The listing builds one solid part. Answer for the finished solid, in the listing's coordinates (mm). Give positions to 0.01 mm unless a question says otherwise; leave off trailing zeros. Loops run counter-clockwise (first coordinate to the right, second up) from the corner with the lowest first, then second, coordinate; pieces in that order, holes last. Notation, with made-up numbers: (51, 25.5) - (78, 25.5) arc R27 cw to (78, 43.5) - close; hole circle Ø1 at (66, 22.25). An arc over 180 degrees is marked (long way). Answer in a Markdown table with one row per item. Add a question column.
```python
from build123d import *

# Parameters (mm, degrees)
SKETCH1_W           = 456
SKETCH1_H           = 626
BASE_FLANGE1_DEPTH  = 1
SKETCH6_W           = 130
SKETCH6_H           = 60
BOSS_EXTRUDE1_DEPTH = 10
SKETCH7_W           = 128
SKETCH7_H           = 58
CUT_EXTRUDE2_DEPTH  = 1
SHELL2_START        = -186
SHELL2_OUTLINE_W    = 58
SHELL2_OUTLINE_H    = 8
SHELL2_DEPTH        = 128
FILLET1_R           = 5


# Read off the part's stored shape, not the designer's step: Shell2
# Sheet-metal steps are written as plain solids
with BuildPart() as part:
    # Sketch1 → Base-Flange1 (new body)
    with BuildSketch(Plane.XY):
        Rectangle(SKETCH1_W, SKETCH1_H)
    extrude(amount=-BASE_FLANGE1_DEPTH)

    # Sketch6 → Boss-Extrude1 (add)
    with BuildSketch(Plane.XY):
        with Locations((-122, 254)):
            Rectangle(SKETCH6_W, SKETCH6_H)
    extrude(amount=-BOSS_EXTRUDE1_DEPTH)

    # Sketch7 → Cut-Extrude2 (cut)
    with BuildSketch(Plane.XY):
        with Locations((-122, 254)):
            Rectangle(SKETCH7_W, SKETCH7_H)
    extrude(amount=-CUT_EXTRUDE2_DEPTH, mode=Mode.SUBTRACT)

    # Shell2 outline → Shell2 (cut)
    with BuildSketch(Plane.YZ.offset(SHELL2_START)):
        with Locations((254, -5)):
            Rectangle(SHELL2_OUTLINE_W, SHELL2_OUTLINE_H)
    extrude(amount=SHELL2_DEPTH, mode=Mode.SUBTRACT)

    # Fillet1
    fillet1_edges = [part.edges().sort_by_distance(p)[0] for p in [
        (-57, 284, -5.5),
        (-57, 224, -5.5),
        (-187, 224, -5.5),
        (-187, 284, -5.5),
        (-186, 225, -4.5),
        (-186, 283, -4.5),
        (-58, 283, -4.5),
        (-58, 225, -4.5),
    ]]
    fillet(fillet1_edges, radius=FILLET1_R)


solid = part.part
```
(1) A cutting plane is placed at B-B on x = -156. Determine the outline of the cut face in (y, z).
(2) Find the intervals of material crossed by line 1 along Y through (x, z) = (-111.5, -2.75); line 2 along X through (y, z) = (268, -1.25); line 3 along Z through (x, y) = (193, 231.5), in increasing order. Write a range as [from, to].
(3) The mould has two halves that part along Y. Classify faces 1 (the face through (-123, 254, -9)), 2 (the face through (-3, 4, 0)): pulls with the +Y half, pulls with the -Y half, needs draft (parallel to the pull), parting line crosses it, or undercut.
(4) A cutting plane is placed at A-A on z = -7.5. Determine the outline of the cut face in (x, y), plus the area to 3 significant figures.
(5) A cutting plane is placed at D-D on x = 197.5. Determine the outline of the cut face in (y, z), plus the area to 3 significant figures.
(6) Given pin 1 Ø4.5 at (y, z) = (246, -5) entering from +X; pin 2 Ø4.5 at (y, z) = (253.5, -7) entering from -X; pin 3 Ø4.5 at (x, z) = (-103.5, -4) entering from +Y; pin 4 Ø1 at (x, y) = (69.5, 229.5) entering from +Z, each flat-ended and moving along its own axis, determine where each tip first touches the part or whether it passes through.
(7) A cutting plane is placed at C-C on y = -155.5. Determine the outline of the cut face in (x, z), plus the area to 3 significant figures.
Evaluation:
| question | item | result |
|---|---|---|
| 1 | outline | (-313, -1) - (224, -1) - (224, -10) - (284, -10) - (284, -1) - (313, -1) - (313, 0) - (283, 0) - (283, -9) - (225, -9) - (225, 0) - (-313, 0) - close |
| 2 | line 1 | y = [224, 225], [283, 284] |
| 2 | line 2 | x = [-187, -186], [-58, -57] |
| 2 | line 3 | z = [-1, 0] |
| 3 | face 1 | undercut |
| 3 | face 2 | needs draft |
| 4 | outline | (-187, 229) arc R5 ccw to (-182, 224) - (-62, 224) arc R5 ccw to (-57, 229) - (-57, 279) arc R5 ccw to (-62, 284) - (-182, 284) arc R5 ccw to (-187, 279) - close; hole (-186, 230) arc R5 ccw to (-181, 225) - (-63, 225) arc R5 ccw to (-58, 230) - (-58, 278) arc R5 ccw to (-63, 283) - (-181, 283) arc R5 ccw to (-186, 278) - close |
| 4 | area | 376 mm² |
| 5 | outline | (-313, -1) - (313, -1) - (313, 0) - (-313, 0) - close |
| 5 | area | 626 mm² |
| 6 | pin 1 | stops at x = -57 |
| 6 | pin 2 | stops at x = -187 |
| 6 | pin 3 | stops at y = 284 |
| 6 | pin 4 | stops at z = 0 |
| 7 | outline | (-228, -1) - (228, -1) - (228, 0) - (-228, 0) - close |
| 7 | area | 456 mm² |
